Print and shaded views of the part. All mm, measured from the part's lowest x, y and z. Round coordinates to 2 decimals unless told otherwise and drop trailing zeros. Write each loop counter-clockwise with the first axis right and the second up, starting at its lowest first coordinate (ties: lowest second). Pieces come first, ordered by that corner, then holes.
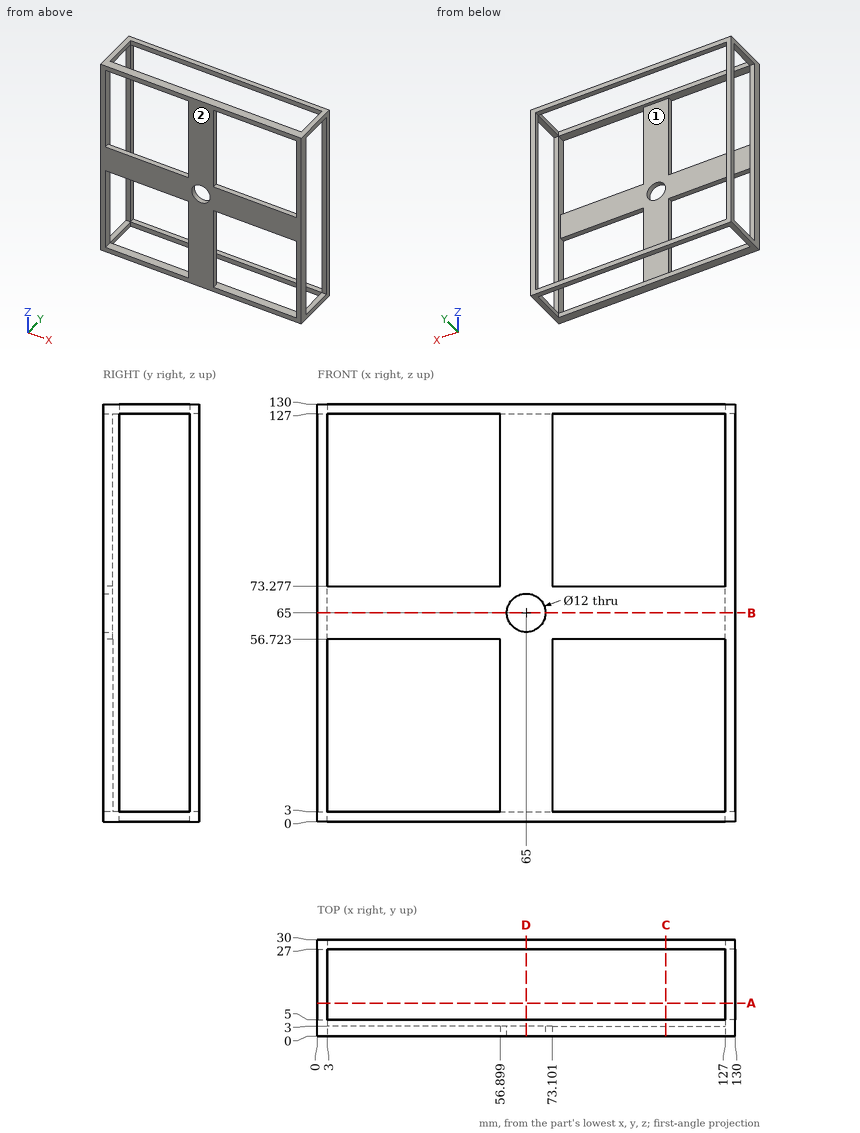
1) Mould opens along Z. For the marked faces 1 and 2 say: released by +Z, released by -Z, zero draft, split by the parting line, or undercut.
Results:
face 1: undercut
face 2: zero draft
2) Slice it at B-B (z = 65). Write the cut outline in (x, y).
Results:
outline: (0, 0) - (59, 0) - (59, 3) - (3, 3) - (3, 5) - (0, 5) - close; (0, 27) - (3, 27) - (3, 30) - (0, 30) - close; (71, 0) - (130, 0) - (130, 5) - (127, 5) - (127, 3) - (71, 3) - close; (127, 27) - (130, 27) - (130, 30) - (127, 30) - close
3) Slice it at A-A (y = 10.25). Write the cut outline in (x, z).
Results:
outline: (0, 0) - (3, 0) - (3, 3) - (0, 3) - close; (0, 127) - (3, 127) - (3, 130) - (0, 130) - close; (127, 0) - (130, 0) - (130, 3) - (127, 3) - close; (127, 127) - (130, 127) - (130, 130) - (127, 130) - close
4) Slice it at C-C (x = 108.5). Write the cut outline in (y, z).
Results:
outline: (0, 0) - (5, 0) - (5, 3) - (0, 3) - close; (0, 56.72) - (3, 56.72) - (3, 73.28) - (0, 73.28) - close; (0, 127) - (5, 127) - (5, 130) - (0, 130) - close; (27, 0) - (30, 0) - (30, 3) - (27, 3) - close; (27, 127) - (30, 127) - (30, 130) - (27, 130) - close
5) Wall check: L1, parallel to X at y = 1.5, z = 65; L2, parallel to X at y = 3.25, z = 104. Give the ranges that are in metal, low to high.
Results:
L1: x = 0 to 59, 71 to 130
L2: x = 0 to 3, 127 to 130
6) Slice it at D-D (x = 65). Write the cut outline in (y, z).
Results:
outline: (0, 0) - (5, 0) - (5, 3) - (3, 3) - (3, 59) - (0, 59) - close; (0, 71) - (3, 71) - (3, 127) - (5, 127) - (5, 130) - (0, 130) - close; (27, 0) - (30, 0) - (30, 3) - (27, 3) - close; (27, 127) - (30, 127) - (30, 130) - (27, 130) - close
7) Pin check, flat tip, straight feed: pin 1 Ø1 at (x, y) = (90.5, 26) entering from +Z. Stop position of the tip, or through.
Results:
pin 1: passes through
